Here's how the part is built. I have some questions about the finished solid (model axes, mm). Face numbers are marked on the shaded views. Coordinates: 2 decimals unless noted, no trailing zeros. Write each loop counter-clockwise with the first axis right and the second up, starting at its lowest first coordinate (ties: lowest second). Pieces come first, ordered by that corner, then holes.
Item 1: If we section it at C-C (x = 0.5): Please give me the cut outline in (y, z).
Item 2: If I drill on line 1 (X direction, y = 10.5, z = 37); line 2 (Y direction, x = 51.5, z = 57.5); line 3 (Y direction, x = 132.9, z = 31.75), over which ranges is the centre line in solid material (lowest first)?
Item 3: I'm going to push flat-ended pins straight in: pin 1 Ø19 at (x, z) = (43, 39) entering from -Y; pin 2 Ø0.5 at (y, z) = (24.5, 14.5) entering from -X; pin 3 Ø1.3 at (y, z) = (24.5, 43.5) entering from -X. Where does each tip first touch, or does it pass through?
Item 4: We'd pull the mould along X, two halves only. Please class the marked faces 1, 2, 3 and 4: +X half, -X half, draft (parallel to the pull), parting line (faces both ways), or undercut.
Item 5: If we section it at B-B (x = -68.5): Please give me the cut outline in (y, z), then the cut area to 3 significant figures.
Item 6: If we section it at A-A (y = 3): Please give me the cut outline in (x, z).
from build123d import *

# Parameters (mm, degrees)
BASE_FLANGE1_DEPTH      = 63.5
CUT_EXTRUDE1_DEPTH      = 276.329439036
CUT_EXTRUDE1_DEPTH_BACK = 276.329439036
SKETCH6_R               = 2.4892
CUT_EXTRUDE2_DEPTH      = 150.865381259
FILLET1_R               = 3.175


# Sheet-metal steps are written as plain solids
with BuildPart() as part:
    # Sketch1 → Base-Flange1 (new body)
    with BuildSketch(Plane.XY):
        with BuildLine():
            Line((-133.35, 0), (-133.35, 23.0505))
            ThreePointArc((-133.35, 23.0505), (-132.661847382, 24.711847382), (-131.0005, 25.4))
            Line((-131.0005, 25.4), (131.0005, 25.4))
            ThreePointArc((131.0005, 25.4), (132.661847382, 24.711847382), (133.35, 23.0505))
            Line((133.35, 23.0505), (133.35, 0))
            Line((133.35, 0), (131.7625, 0))
            Line((131.7625, 0), (131.7625, 23.0505))
            ThreePointArc((131.7625, 23.0505), (131.539315367, 23.589315367), (131.0005, 23.8125))
            Line((131.0005, 23.8125), (-131.0005, 23.8125))
            ThreePointArc((-131.0005, 23.8125), (-131.539315367, 23.589315367), (-131.7625, 23.0505))
            Line((-131.7625, 23.0505), (-131.7625, 0))
            Line((-131.7625, 0), (-133.35, 0))
        make_face()
    extrude(amount=BASE_FLANGE1_DEPTH)

    # Sketch6 → Cut-Extrude1 (cut, two sides: drawn at the far end of the back side and taken through both)
    with BuildSketch(Plane.ZY.offset(133.35).offset(-CUT_EXTRUDE1_DEPTH_BACK)):
        with Locations((12.7, 11.52525)):
            Circle(SKETCH6_R)
        with Locations((50.8, 11.52525)):
            Circle(SKETCH6_R)
        with Locations((31.75, 11.52525)):
            Circle(SKETCH6_R)
    extrude(amount=CUT_EXTRUDE1_DEPTH + CUT_EXTRUDE1_DEPTH_BACK, mode=Mode.SUBTRACT)

    # Sketch7 → Cut-Extrude2 (cut, through all)
    with BuildSketch(Plane(origin=(0, 25.4, 0), x_dir=(1, 0, 0), z_dir=(0, 1, 0))):
        Polygon((-104.775, -42.468871356), (-104.775, -6.35), (-121.163937878, -6.35), align=None)
        Polygon((-124.6505, -57.15), (-105.086562122, -57.15), (-124.6505, -14.033883464), align=None)
        Polygon((-98.425, -49.484871939), (-55.290128061, -6.35), (-98.425, -6.35), align=None)
        Polygon((-97.109871939, -57.15), (-53.975, -57.15), (-53.975, -14.015128061), align=None)
        Polygon((-47.625, -57.15), (-4.490128061, -57.15), (-47.625, -14.015128061), align=None)
        Polygon((-3.175, -49.484871939), (-3.175, -6.35), (-46.309871939, -6.35), align=None)
        Polygon((3.175, -49.484871939), (46.309871939, -6.35), (3.175, -6.35), align=None)
        Polygon((4.490128061, -57.15), (47.625, -57.15), (47.625, -14.015128061), align=None)
        Polygon((105.086562122, -57.15), (124.6505, -57.15), (124.6505, -14.033883464), align=None)
        Polygon((104.775, -42.468871356), (121.163937878, -6.35), (104.775, -6.35), align=None)
        Polygon((55.290128061, -6.35), (98.425, -49.484871939), (98.425, -6.35), align=None)
        Polygon((53.975, -57.15), (97.109871939, -57.15), (53.975, -14.015128061), align=None)
    extrude(amount=-CUT_EXTRUDE2_DEPTH, mode=Mode.SUBTRACT)

    # Fillet1
    fillet1_edges = [part.edges().sort_by_distance(p)[0] for p in [
        (-3.175, 24.60625, 6.35),
        (-3.175, 24.60625, 49.484871939),
        (-46.309871939, 24.60625, 6.35),
        (3.175, 24.60625, 6.35),
        (46.309871939, 24.60625, 6.35),
        (3.175, 24.60625, 49.484871939),
        (47.625, 24.60625, 14.015128061),
        (47.625, 24.60625, 57.15),
        (4.490128061, 24.60625, 57.15),
        (124.6505, 24.60625, 14.033883464),
        (124.6505, 24.60625, 57.15),
        (105.086562122, 24.60625, 57.15),
        (-105.086562122, 24.60625, 57.15),
        (-124.6505, 24.60625, 57.15),
        (-124.6505, 24.60625, 14.033883464),
        (-55.290128061, 24.60625, 6.35),
        (-98.425, 24.60625, 49.484871939),
        (-98.425, 24.60625, 6.35),
        (-53.975, 24.60625, 14.015128061),
        (-53.975, 24.60625, 57.15),
        (-97.109871939, 24.60625, 57.15),
        (-4.490128061, 24.60625, 57.15),
        (-47.625, 24.60625, 57.15),
        (-47.625, 24.60625, 14.015128061),
        (53.975, 24.60625, 14.015128061),
        (97.109871939, 24.60625, 57.15),
        (53.975, 24.60625, 57.15),
        (98.425, 24.60625, 49.484871939),
        (55.290128061, 24.60625, 6.35),
        (98.425, 24.60625, 6.35),
        (121.163937878, 24.60625, 6.35),
        (104.775, 24.60625, 42.468871356),
        (104.775, 24.60625, 6.35),
        (-104.775, 24.60625, 42.468871356),
        (-121.163937878, 24.60625, 6.35),
        (-104.775, 24.60625, 6.35),
    ]]
    fillet(fillet1_edges, radius=FILLET1_R)


solid = part.part
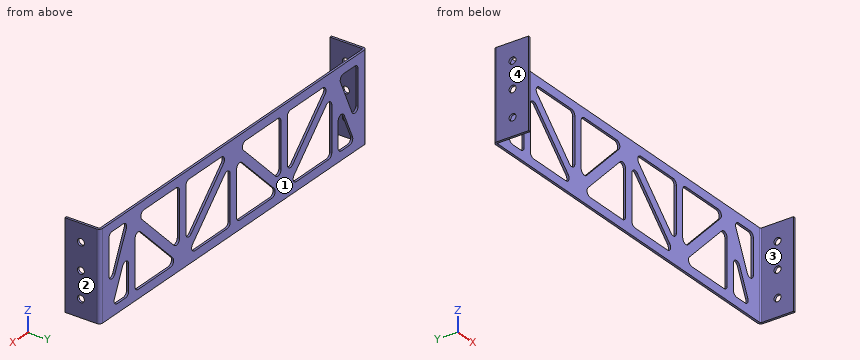
Answer list:
1. outline: (23.81, 0) - (25.4, 0) - (25.4, 63.5) - (23.81, 63.5) - close
2. line 1: x = -133.35 to -131.76, 131.76 to 133.35
2. line 2: y = 23.81 to 25.4
2. line 3: y = 0 to 9.04, 14.01 to 24.43
3. pin 1: stops at y = 23.81
3. pin 2: stops at x = -133.02
3. pin 3: stops at x = -133.21
4. face 1: draft
4. face 2: +X half
4. face 3: undercut
4. face 4: -X half
5. outline: (23.81, 0) - (25.4, 0) - (25.4, 6.35) - (23.81, 6.35) - close; (23.81, 19.56) - (25.4, 19.56) - (25.4, 28.54) - (23.81, 28.54) - close; (23.81, 57.15) - (25.4, 57.15) - (25.4, 63.5) - (23.81, 63.5) - close
5. area: 34.4 mm2
6. outline: (-133.35, 0) - (-131.76, 0) - (-131.76, 63.5) - (-133.35, 63.5) - close; (131.76, 0) - (133.35, 0) - (133.35, 63.5) - (131.76, 63.5) - close
